Read the model definition and answer for the solid it produces. Units are mm, in the model's axes. A direction names the side the tool comes from. Coordinates: 2 decimals unless noted, no trailing zeros. Order: outer loops, then holes, each group sorted by start corner. A loop starts at its lowest first (then second) coordinate and runs counter-clockwise, first axis right, second up. Notation, with made-up numbers: (-11.5, 7.5) -> (-2.5, 7.5) arc R32 ccw to (-2.5, 39.5) -> close; hole circle Ø4 at (-14.5, -11). An arc over 180 degrees is marked (long way). Answer as a JSON object with one key per item and string values. Group by question number.
1) Consider L1, parallel to Z at x = 43, y = 2.25; L2, parallel to Z at x = -44, y = 4.5; L3, parallel to Z at x = 1, y = 7. Determine where each line is inside the solid, lowest interval first.
2) Determine the mould class of faces 4 (the flat face through (-27, 5, -27.851)), 5 (the cylindrical face through (-9.65, 5.07, -64.84)) for opening direction X: released by +X, released by -X, zero draft, split by the parting line, or undercut.
3) Section B-B on z = -50.5 is taken. Determine the outline of the cut face in (x, y).
4) Section C-C on y = 5.5 is taken. Count the separate pieces of the cut face and the enclosed holes in it, and give its area (3 significant figures).
5) A tool of negligible diameter and unlimited length cuts with its end or side. For faces 1 (the flat face through (-2.5, 5, -53)), 2 (the flat face through (-30, 5, -37.851)), 3 (the flat face through (-62.5, 5, 30)), from which of +Z, -Z, +X, -X, +Y, -Y can it reach the whole face along a straight path? Write none if from no direction.
6) Given pin 1 (6 mm diameter, centred on y = 3.5, z = -45, fed in from -X); pin 2 (2 mm diameter, centred on x = -10, y = 4.5, fed in from +Z); pin 3 (3 mm diameter, centred on y = 7.5, z = -2, fed in from -X), each flat-ended and moving along its own axis, determine where each tip first touches the part or whether it passes through.
7) Section A-A on x = -27.5 is taken. Determine the outline of the cut face in (y, z), and give its area (3 significant figures).
from build123d import *

# Parameters (mm, degrees)
BOSS_EXTRUDE1_DEPTH = 10
FILLET1_R           = 10
FILLET2_R           = 10
FILLET3_R           = 10
CUT_EXTRUDE1_DEPTH  = 10
CUT_EXTRUDE2_DEPTH  = 10
SKETCH5_R           = 5.34535751
BOSS_EXTRUDE2_DEPTH = 10
SKETCH7_R           = 2.1
CUT_EXTRUDE3_DEPTH  = 10
SKETCH13_R          = 2.1
CUT_EXTRUDE4_DEPTH  = 10
SKETCH15_W          = 75
SKETCH15_H          = 10
BOSS_EXTRUDE3_DEPTH = 10
SKETCH18_W          = 60
SKETCH18_H          = 10
BOSS_EXTRUDE4_DEPTH = 10
SKETCH19_R          = 2.4
SKETCH19_R_2        = 2.8
CUT_EXTRUDE6_DEPTH  = 10
SKETCH20_W          = 80
SKETCH20_H          = 10
BOSS_EXTRUDE5_DEPTH = 10
CUT_EXTRUDE7_DEPTH  = 10
FILLET4_R           = 10
SKETCH22_W          = 10
SKETCH22_H          = 20
CUT_EXTRUDE8_DEPTH  = 10
FILLET5_START       = -1
FILLET5_DEPTH       = 12
FILLET5_2_DEPTH     = 10
SKETCH24_W          = 15
SKETCH24_H          = 10
BOSS_EXTRUDE6_DEPTH = 5
SKETCH25_W          = 15
SKETCH25_H          = 10
BOSS_EXTRUDE7_DEPTH = 5
SKETCH26_R          = 2.5
CUT_EXTRUDE9_DEPTH  = 15
FILLET6_R           = 5


with BuildPart() as part:
    # Sketch1 → Boss-Extrude1 (new body)
    with BuildSketch(Plane(origin=(0, 0, 0), x_dir=(1, 0, 0), z_dir=(0, 1, 0))):
        Polygon((-52.5, 37.850859258), (-12.5, 37.850859258), (-12.5, 67.850859258), (52.5, 67.850859258), (52.5, -72.149140742), (-12.5, -72.149140742), (-12.5, -42.149140742), (-52.5, -42.149140742), align=None)
    extrude(amount=BOSS_EXTRUDE1_DEPTH)

    # Fillet1
    fillet1_edges = [part.edges().sort_by_distance(p)[0] for p in [
        (-12.5, 5, 42.149140742),
        (-12.5, 5, -37.850859258),
    ]]
    fillet(fillet1_edges, radius=FILLET1_R)

    # Fillet2
    fillet2_edges = [part.edges().sort_by_distance(p)[0] for p in [
        (-12.5, 5, 72.149140742),
        (-12.5, 5, -67.850859258),
    ]]
    fillet(fillet2_edges, radius=FILLET2_R)

    # Fillet3
    fillet3_edges = [part.edges().sort_by_distance(p)[0] for p in [
        (52.5, 5, 72.149140742),
        (52.5, 5, -67.850859258),
    ]]
    fillet(fillet3_edges, radius=FILLET3_R)

    # Sketch3 → Cut-Extrude1 (cut)
    with BuildSketch(Plane(origin=(0, 10, 0), x_dir=(1, 0, 0), z_dir=(0, 1, 0))):
        with BuildLine():
            ThreePointArc((51, 43.850859258), (48.51040764, 49.861266898), (42.5, 52.350859258))
            Line((42.5, 52.350859258), (42.5, 35.350859258))
            ThreePointArc((42.5, 35.350859258), (48.51040764, 37.840451618), (51, 43.850859258))
        make_face()
        with BuildLine():
            Line((42.5, 35.350859258), (42.5, 52.350859258))
            ThreePointArc((42.5, 52.350859258), (34, 43.850859258), (42.5, 35.350859258))
        make_face()
        with BuildLine():
            ThreePointArc((51, -48.149140742), (48.51040764, -42.138733102), (42.5, -39.649140742))
            Line((42.5, -39.649140742), (42.5, -56.649140742))
            ThreePointArc((42.5, -56.649140742), (48.51040764, -54.159548382), (51, -48.149140742))
        make_face()
        with BuildLine():
            Line((42.5, -56.649140742), (42.5, -39.649140742))
            ThreePointArc((42.5, -39.649140742), (34, -48.149140742), (42.5, -56.649140742))
        make_face()
    extrude(amount=-CUT_EXTRUDE1_DEPTH, mode=Mode.SUBTRACT)

    # Sketch4 → Cut-Extrude2 (cut)
    with BuildSketch(Plane(origin=(0, 10, 0), x_dir=(1, 0, 0), z_dir=(0, 1, 0))):
        with BuildLine():
            Line((-2.5, -62.149140742), (42.5, -62.149140742))
            Line((42.5, -62.149140742), (42.5, 57.850859258))
            Line((42.5, 57.850859258), (-2.5, 57.850859258))
            Line((-2.5, 57.850859258), (-2.5, 47.850859258))
            ThreePointArc((-2.5, 47.850859258), (-8.357864376, 33.708723634), (-22.5, 27.850859258))
            Line((-22.5, 27.850859258), (-42.5, 27.850859258))
            Line((-42.5, 27.850859258), (-42.5, -32.149140742))
            Line((-42.5, -32.149140742), (-22.5, -32.149140742))
            ThreePointArc((-22.5, -32.149140742), (-8.357864376, -38.007005118), (-2.5, -52.149140742))
            Line((-2.5, -52.149140742), (-2.5, -62.149140742))
        make_face()
    extrude(amount=-CUT_EXTRUDE2_DEPTH, mode=Mode.SUBTRACT)

    # Sketch5 → Boss-Extrude2 (add)
    with BuildSketch(Plane(origin=(0, 10, 0), x_dir=(1, 0, 0), z_dir=(0, 1, 0))):
        with Locations((12.473028737, 59.850859258)):
            Circle(SKETCH5_R)
        with Locations((12.473028737, -64.149140742)):
            Circle(SKETCH5_R)
    extrude(amount=-BOSS_EXTRUDE2_DEPTH)

    # Sketch7 → Cut-Extrude3 (cut)
    with BuildSketch(Plane(origin=(0, 10, 0), x_dir=(1, 0, 0), z_dir=(0, 1, 0))):
        with Locations(Location((12.473028737, 59.850859258, 0), (0, 0, 270))):
            Circle(SKETCH7_R)
        with Locations(Location((12.473028737, -64.149140742, 0), (0, 0, 270))):
            Circle(SKETCH7_R)
    extrude(amount=-CUT_EXTRUDE3_DEPTH, mode=Mode.SUBTRACT)

    # Sketch13 → Cut-Extrude4 (cut)
    with BuildSketch(Plane(origin=(0, 10, 0), x_dir=(1, 0, 0), z_dir=(0, 1, 0))):
        with Locations(Location((-35.553942525, -35.649140742, 0), (0, 0, 270))):
            Circle(SKETCH13_R)
        with Locations(Location((-35.553942525, 31.350859258, 0), (0, 0, 270))):
            Circle(SKETCH13_R)
    extrude(amount=-CUT_EXTRUDE4_DEPTH, mode=Mode.SUBTRACT)

    # Sketch15 → Boss-Extrude3 (add)
    with BuildSketch(Plane.ZY.offset(-42.5)):
        with Locations((2.149140742, 5)):
            Rectangle(SKETCH15_W, SKETCH15_H)
    extrude(amount=BOSS_EXTRUDE3_DEPTH)

    # Sketch18 → Boss-Extrude4 (add)
    with BuildSketch(Plane(origin=(-42.5, 0, 0), x_dir=(0, 0, -1), z_dir=(1, 0, 0))):
        with Locations((-2.149140742, 5)):
            Rectangle(SKETCH18_W, SKETCH18_H)
    extrude(amount=BOSS_EXTRUDE4_DEPTH)

    # Sketch19 → Cut-Extrude6 (cut)
    with BuildSketch(Plane(origin=(0, 10, 0), x_dir=(1, 0, 0), z_dir=(0, 1, 0))):
        with Locations(Location((-45.5, 28.502344732, 0), (0, 0, 270))):
            Circle(SKETCH19_R)
        with Locations(Location((-45.5, -32.57798884, 0), (0, 0, 270))):
            Circle(SKETCH19_R)
        with Locations(Location((44.5, -32.342002638, 0), (0, 0, 270))):
            Circle(SKETCH19_R_2)
        with Locations(Location((44.5, 28.502344732, 0), (0, 0, 270))):
            Circle(SKETCH19_R_2)
    extrude(amount=-CUT_EXTRUDE6_DEPTH, mode=Mode.SUBTRACT)

    # Sketch20 → Boss-Extrude5 (add)
    with BuildSketch(Plane.ZY.offset(52.5)):
        with Locations((2.149140742, 5)):
            Rectangle(SKETCH20_W, SKETCH20_H)
    extrude(amount=BOSS_EXTRUDE5_DEPTH)

    # Sketch21 → Cut-Extrude7 (cut)
    with BuildSketch(Plane(origin=(0, 10, 0), x_dir=(1, 0, 0), z_dir=(0, 1, 0))):
        with BuildLine():
            ThreePointArc((-54.5, 22.850859258), (-55.378679656, 24.972179602), (-57.5, 25.850859258))
            Line((-57.5, 25.850859258), (-57.5, 19.850859258))
            ThreePointArc((-57.5, 19.850859258), (-55.378679656, 20.729538915), (-54.5, 22.850859258))
        make_face()
        with BuildLine():
            Line((-57.5, 19.850859258), (-57.5, 25.850859258))
            ThreePointArc((-57.5, 25.850859258), (-60.5, 22.850859258), (-57.5, 19.850859258))
        make_face()
        with BuildLine():
            ThreePointArc((-54.5, -27.149140742), (-55.378679656, -25.027820398), (-57.5, -24.149140742))
            Line((-57.5, -24.149140742), (-57.5, -30.149140742))
            ThreePointArc((-57.5, -30.149140742), (-55.378679656, -29.270461085), (-54.5, -27.149140742))
        make_face()
        with BuildLine():
            Line((-57.5, -30.149140742), (-57.5, -24.149140742))
            ThreePointArc((-57.5, -24.149140742), (-60.5, -27.149140742), (-57.5, -30.149140742))
        make_face()
    extrude(amount=-CUT_EXTRUDE7_DEPTH, mode=Mode.SUBTRACT)

    # Fillet4
    fillet4_edges = [part.edges().sort_by_distance(p)[0] for p in [
        (-62.5, 5, -37.850859258),
        (-62.5, 5, 42.149140742),
    ]]
    fillet(fillet4_edges, radius=FILLET4_R)

    # Sketch22 → Cut-Extrude8 (cut)
    with BuildSketch(Plane(origin=(0, 10, 0), x_dir=(1, 0, 0), z_dir=(0, 1, 0))):
        with Locations((-57.5, 7.850859258)):
            Rectangle(SKETCH22_W, SKETCH22_H)
        with Locations((-57.5, -12.149140742)):
            Rectangle(SKETCH22_W, SKETCH22_H)
    extrude(amount=-CUT_EXTRUDE8_DEPTH, mode=Mode.SUBTRACT)

    # Fillet5: read off the stored shape, not the designer's step
    # Fillet5 outline → Fillet5 (cut)
    with BuildSketch(Plane(origin=(0, 0, 0), x_dir=(1, 0, 0), z_dir=(0, 1, 0)).offset(FILLET5_START)):
        with BuildLine():
            Line((-62.5, 17.850859258), (-57.5, 17.850859258))
            ThreePointArc((-57.5, 17.850859258), (-61.035533906, 19.315325352), (-62.5, 22.850859258))
            Line((-62.5, 22.850859258), (-62.5, 17.850859258))
        make_face()
        with BuildLine():
            ThreePointArc((-62.5, -27.149140742), (-61.035533906, -23.613606836), (-57.5, -22.149140742))
            Line((-57.5, -22.149140742), (-62.5, -22.149140742))
            Line((-62.5, -22.149140742), (-62.5, -27.149140742))
        make_face()
    extrude(amount=FILLET5_DEPTH, mode=Mode.SUBTRACT)

    # Fillet5 2 outline → Fillet5 2 (add)
    with BuildSketch(Plane(origin=(0, 0, 0), x_dir=(1, 0, 0), z_dir=(0, 1, 0))):
        with BuildLine():
            Line((-52.5, 17.850859258), (-57.5, 17.850859258))
            ThreePointArc((-57.5, 17.850859258), (-53.964466094, 16.386393164), (-52.5, 12.850859258))
            Line((-52.5, 12.850859258), (-52.5, 17.850859258))
        make_face()
        with BuildLine():
            Line((-52.5, -22.149140742), (-52.5, -17.149140742))
            ThreePointArc((-52.5, -17.149140742), (-53.964466094, -20.684674648), (-57.5, -22.149140742))
            Line((-57.5, -22.149140742), (-52.5, -22.149140742))
        make_face()
    extrude(amount=FILLET5_2_DEPTH)

    # Sketch24 → Boss-Extrude6 (add)
    with BuildSketch(Plane.XY.offset(42.149140742)):
        with Locations((-45, 5)):
            Rectangle(SKETCH24_W, SKETCH24_H)
    extrude(amount=BOSS_EXTRUDE6_DEPTH)

    # Sketch25 → Boss-Extrude7 (add)
    with BuildSketch(Plane(origin=(0, 0, -37.850859258), x_dir=(-1, 0, 0), z_dir=(0, 0, -1))):
        with Locations((45, 5)):
            Rectangle(SKETCH25_W, SKETCH25_H)
    extrude(amount=BOSS_EXTRUDE7_DEPTH)

    # Sketch26 → Cut-Extrude9 (cut)
    with BuildSketch(Plane(origin=(0, 10, 0), x_dir=(1, 0, 0), z_dir=(0, 1, 0))):
        with Locations(Location((-45.25, 17.408381721, 0), (0, 0, 270))):
            Circle(SKETCH26_R)
        with Locations(Location((-45.25, -40.591618279, 0), (0, 0, 270))):
            Circle(SKETCH26_R)
        with Locations((43.75, -40.591618279)):
            Circle(SKETCH26_R)
        with Locations(Location((43.75, 17.408381721, 0), (0, 0, 270))):
            Circle(SKETCH26_R)
    extrude(amount=-CUT_EXTRUDE9_DEPTH, mode=Mode.SUBTRACT)

    # Fillet6
    fillet6_edges = [part.edges().sort_by_distance(p)[0] for p in [
        (-37.5, 5, 47.149140742),
        (-37.5, 5, -42.850859258),
        (-52.5, 5, -42.850859258),
        (-52.5, 5, 47.149140742),
    ]]
    fillet(fillet6_edges, radius=FILLET6_R - 0.0001)  # a hair under: the kernel refuses the full size


solid = part.part
Worked answers:
{
 "1": {"L1": "z = -67.84 to -52.34, -35.37 to -30.87, -26.14 to -19.79, -15.02 to 29.98, 34.71 to 38.21, 56.63 to 72.14", "L2": "z = -42.85 to -30.38, -26.63 to -19.57, -15.24 to 30.7, 34.45 to 38.43, 42.76 to 47.15", "L3": "z = -67.85 to -57.85, 62.15 to 72.15"},
 "2": {"face 4": "undercut", "face 5": "released by -X"},
 "3": {"outline": "(-12.5, 0) -> (-2.5, 0) -> (-2.5, 10) -> (-12.5, 10) -> close; (47.8, 0) -> (52.5, 0) -> (52.5, 10) -> (47.8, 10) -> close"},
 "4": {"separate pieces": "1", "enclosed holes": "14", "area": "5,680 mm²"},
 "5": {"face 1": "+Y, -Y", "face 2": "-Z, +Y, -Y", "face 3": "+Z, -Z, -X, +Y, -Y"},
 "6": {"pin 1": "stops at x = -50.29", "pin 2": "stops at z = 69.75", "pin 3": "stops at x = -52.5"},
 "7": {"outline": "(0, -37.85) -> (10, -37.85) -> (10, -27.85) -> (0, -27.85) -> close; (0, 32.15) -> (10, 32.15) -> (10, 42.15) -> (0, 42.15) -> close", "area": "200 mm²"}
}
